Source: CAD feature listing. Evaluate the final solid. Frame: model axes, mm. A direction names the side the tool comes from. Give positions to 0.01 mm unless a question says otherwise; leave off trailing zeros. Loops run counter-clockwise (first coordinate to the right, second up) from the corner with the lowest first, then second, coordinate; pieces in that order, holes last. Notation, with made-up numbers: (22.25, 15) -> (59.25, 15) arc R22 cw to (59.25, 28) -> close; hole circle Ø2 at (-33.5, 41). An arc over 180 degrees is marked (long way). Return JSON: item names as keys, results as strings. Group by question number.
```python
from build123d import *

# Parameters (mm, degrees)
BOSS_EXTRUDE1_DEPTH = 4
FILLET1_R           = 1
SKETCH4_W           = 17.5
SKETCH4_H           = 17.5
BOSS_EXTRUDE3_DEPTH = 5


with BuildPart() as part:
    # Sketch2 → Boss-Extrude1 (new body)
    with BuildSketch(Plane(origin=(0, 0, 0), x_dir=(1, 0, 0), z_dir=(0, 1, 0))):
        Polygon((0, 0), (26.5, 0), (26.5, -26), (28.5, -26), (28.5, 0), (30, 0), (30, 13.5), (57, 13.5), (57, 15.5), (29, 15.5), (27.5, 15.5), (27.5, 17.5), (2.991015417, 17.5), (-11.508984583, 17.5), (-11.508984583, 0), align=None)
    extrude(amount=BOSS_EXTRUDE1_DEPTH)

    # Fillet1
    fillet1_edges = [part.edges().sort_by_distance(p)[0] for p in [
        (42.25, 0, -15.5),
        (28.5, 0, 13),
        (26.5, 0, 13),
        (43.5, 0, -13.5),
        (42.25, 4, -15.5),
        (43.5, 4, -13.5),
        (28.5, 4, 13),
        (26.5, 4, 13),
    ]]
    fillet(fillet1_edges, radius=FILLET1_R - 0.0001)  # a hair under: the kernel refuses the full size

    # Sketch4 → Boss-Extrude3 (add)
    with BuildSketch(Plane(origin=(0, 4, 0), x_dir=(1, 0, 0), z_dir=(0, 1, 0))):
        with Locations((-2.758984583, 8.75)):
            Rectangle(SKETCH4_W, SKETCH4_H)
    extrude(amount=BOSS_EXTRUDE3_DEPTH)


solid = part.part
```
1) Contact query for flat-ended pins moving along their axis: P1, Ø5, axis at x = 46.5, z = -12, coming from the +Y side; P2, Ø1, axis at x = 36.5, y = 1.5, coming from the -Z side; P3, Ø1.6, axis at y = 2, z = 14, coming from the +X side. Output: stop coordinate, or through.
2) Reachability of faces 1 (the face through (7, 0, -7)), 2 (the face through (42, 2, -15.5)), 3 (the face through (18, 4, -9)), 4 (the face through (43, 2, -13.5)), 5 (the face through (26.5, 2, 13)) from +Z, -Z, +X, -X, +Y, -Y: full face, straight path, thin tool, end or side. Return the list, or none.
3) Cut plane A-A on y = 2. Return loops of the section in (x, z).
4) Cut plane D-D on y = 5.5. Return loops of the section in (x, z), then the cut area to 3 significant figures.
5) Material intervals for line 1 (X direction, y = 6.5, z = -3); line 2 (X direction, y = 3.75, z = -8.5); line 3 (Z direction, x = 1.5, y = 4.5), sorted ascending.
Calculated:
{
 "1": {"P1": "y = 4", "P2": "z = -15.5", "P3": "x = 28.5"},
 "2": {"face 1": "+Z, -Z, +X, -X, -Y", "face 2": "-Z, +X, +Y, -Y", "face 3": "+Z, -Z, +X, +Y", "face 4": "+Z, +X, +Y, -Y", "face 5": "+Z, -X, +Y, -Y"},
 "3": {"outline": "(-11.51, -17.5) -> (27.5, -17.5) -> (27.5, -15.5) -> (57, -15.5) -> (57, -13.5) -> (30, -13.5) -> (30, 0) -> (28.5, 0) -> (28.5, 26) -> (26.5, 26) -> (26.5, 0) -> (-11.51, 0) -> close"},
 "4": {"outline": "(-11.51, -17.5) -> (5.99, -17.5) -> (5.99, 0) -> (-11.51, 0) -> close", "area": "306 mm2"},
 "5": {"line 1": "-11.51 to 5.99", "line 2": "-11.51 to 30", "line 3": "-17.5 to 0"}
}
